Check sheet for the drawn part. Datum: minimum x, y, z corner. Units: mm. A direction names the side the tool comes from. Round coordinates to 2 decimals unless told otherwise and drop trailing zeros. Write each loop counter-clockwise with the first axis right and the second up, starting at its lowest first coordinate (ties: lowest second). Pieces come first, ordered by that corner, then holes.
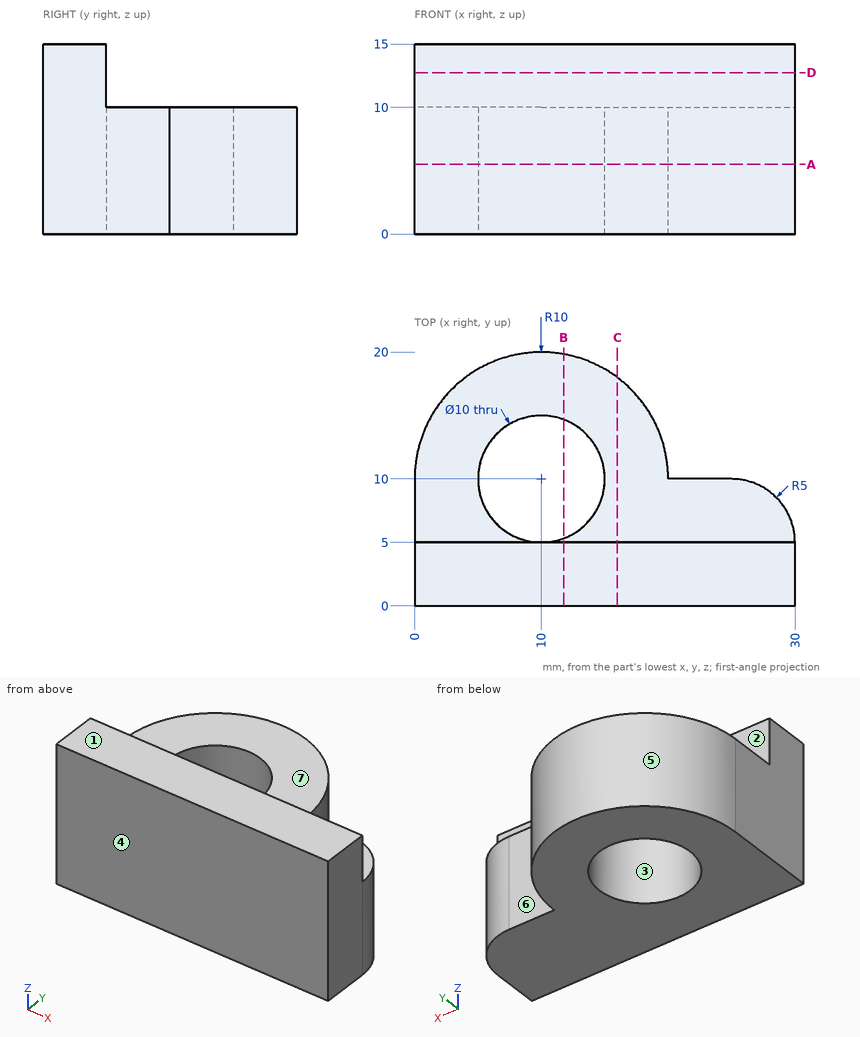
Q1. Material ranges on line 1 along Y through (x, z) = (10, 8); line 2 along Z through (x, y) = (4.25, 14); line 3 along X through (y, z) = (11.25, 2.5), recorded low to high.
Recorded:
line 1: y = 0 to 5, 15 to 20
line 2: z = 0 to 10
line 3: x = 0.08 to 5.16, 14.84 to 19.92
Q2. Depth check by flat-ended pin: P1, Ø8, axis at x = 18.5, y = 3.5, coming from the -Z side; P2, Ø3, axis at x = 24, z = 7, coming from the +Y side; P3, Ø4, axis at y = 14, z = 8.5, coming from the -X side. Enter the tip coordinate at first touch or a pass-through.
Recorded:
P1: stops at z = 0
P2: stops at y = 10
P3: stops at x = 0.2
Q3. Release check for a two-part mould opening along Y. For the marked faces 1, 2, 3 and 4 record: released by +Y, released by -Y, zero draft, split by the parting line, or undercut.
Recorded:
face 1: zero draft
face 2: released by +Y
face 3: undercut
face 4: released by -Y
Q4. Sectioned sample at A-A (z = 5.5). Enter the section's corners in (x, y).
Recorded:
outline: (0, 0) - (30, 0) - (30, 5) arc R5 ccw to (25, 10) - (20, 10) arc R10 ccw to (0, 10) - close; hole circle Ø10 at (10, 10)
Q5. Sectioned sample at D-D (z = 12.75). Enter the section's corners in (x, y), plus the area to 3 significant figures.
Recorded:
outline: (0, 0) - (30, 0) - (30, 5) - (0, 5) - close
area: 150 mm2
Q6. Sectioned sample at B-B (x = 11.75). Enter the section's corners in (y, z).
Recorded:
outline: (0, 0) - (5.32, 0) - (5.32, 10) - (5, 10) - (5, 15) - (0, 15) - close; (14.68, 0) - (19.85, 0) - (19.85, 10) - (14.68, 10) - close
Q7. Tool access check on the marked faces 5, 6 and 7. Record the directions out of +Z, -Z, +X, -X, +Y, -Y that give a thin tool (end or side, any length) a straight path to the whole face; none if there is none.
Recorded:
face 5: +Z, -Z, +Y
face 6: +Z, -Z, +X, +Y
face 7: +Z, +X, -X, +Y
Q8. Sectioned sample at C-C (x = 16). Enter the section's corners in (y, z), plus the area to 3 significant figures.
Recorded:
outline: (0, 0) - (18, 0) - (18, 10) - (5, 10) - (5, 15) - (0, 15) - close
area: 205 mm2
